Input: part model. Units: mm. Frame: model coordinates. Round coordinates to 2 decimals unless told otherwise and drop trailing zeros. Write each loop counter-clockwise with the first axis right and the second up, starting at its lowest first coordinate (ties: lowest second). Pieces come first, ordered by that corner, then holes. Notation, with made-up numbers: (-31, 52.25) - (11, 52.25) arc R18 ccw to (11, 71.25) - close; hole circle Ø5 at (-27.75, 23.25). An arc over 180 degrees is marked (long way). Use one line per item in the form item = value.
```python
from build123d import *

# Parameters (mm, degrees)
SKETCH_W        = 110
SKETCH_H        = 80
PAD_DEPTH       = 6
SKETCH001_R     = 1.4
POCKET_DEPTH    = 8
SKETCH002_R     = 2
POCKET001_DEPTH = 6


with BuildPart() as part:
    # Sketch → Pad (new body)
    with BuildSketch(Plane.XY):
        Rectangle(SKETCH_W, SKETCH_H)
    extrude(amount=PAD_DEPTH)

    # Sketch001 → Pocket (cut)
    with BuildSketch(Plane.XY.offset(6)):
        with Locations((-38.660252, 15)):
            Circle(SKETCH001_R)
        with Locations((-21.339748, -15)):
            Circle(SKETCH001_R)
        with Locations((-8.660252, 15)):
            Circle(SKETCH001_R)
        with Locations((8.660252, -15)):
            Circle(SKETCH001_R)
        with Locations((21.339748, 15)):
            Circle(SKETCH001_R)
        with Locations((38.660252, -15)):
            Circle(SKETCH001_R)
    extrude(amount=-POCKET_DEPTH, mode=Mode.SUBTRACT)

    # Sketch002 → Pocket001 (cut)
    with BuildSketch(Plane.XY.offset(6)):
        with Locations((-44.5, 32.1)):
            Circle(SKETCH002_R)
        with Locations((38.4, 32.1)):
            Circle(SKETCH002_R)
        with Locations((-30.4, 32.1)):
            Circle(SKETCH002_R)
        with Locations((-10.1, 32.1)):
            Circle(SKETCH002_R)
        with Locations((24.3, 32.1)):
            Circle(SKETCH002_R)
        with Locations((4, 32.1)):
            Circle(SKETCH002_R)
    pocket001 = extrude(amount=-POCKET001_DEPTH, mode=Mode.SUBTRACT)

    # Mirrored: Pocket001 across Sketch002 H_Axis
    add(pocket001.mirror(Plane(origin=(0, 0, 6), x_dir=(0, 0, 1), z_dir=(0, 1, 0))), mode=Mode.SUBTRACT)


solid = part.part
```
(1) Cut plane C-C on z = 3.4. Count the separate pieces of the cut face and the enclosed holes in it, then the cut area to 3 significant figures.
Derived:
separate_pieces = 1
enclosed_holes = 18
area = 8,610 mm^2
(2) Cut plane A-A on y = -15. Output: boundary loops of the cut face in (x, z).
Derived:
outline = (-55, 0) - (-22.74, 0) - (-22.74, 6) - (-55, 6) - close; (-19.94, 0) - (7.26, 0) - (7.26, 6) - (-19.94, 6) - close; (10.06, 0) - (37.26, 0) - (37.26, 6) - (10.06, 6) - close; (40.06, 0) - (55, 0) - (55, 6) - (40.06, 6) - close
(3) Material intervals for L1, parallel to Y at x = 38.4, z = 3.3; L2, parallel to Y at x = -44.5, z = 3.95; L3, parallel to Y at x = -43, z = 4.8, sorted ascending.
Derived:
L1 = -40 to -34.1, -30.1 to -16.38, -13.62 to 30.1, 34.1 to 40
L2 = -40 to -34.1, -30.1 to 30.1, 34.1 to 40
L3 = -40 to -33.42, -30.78 to 30.78, 33.42 to 40
(4) First-contact query: pin 1 Ø3.5 at (x, y) = (4, -32.1) entering from -Z. Flat tip, straight axial feed; report the tip coordinate or a pass-through.
Derived:
pin_1 = through
(5) Draft query along X for faces 1 (the face through (-55, -1, 3)), 2 (the face through (-1, 40, 3)), 3 (the face through (22.302, 32.188, 3.042)). Return one class per face: released by +X, released by -X, zero draft, split by the parting line, or undercut.
Derived:
face_1 = released by -X
face_2 = zero draft
face_3 = undercut
(6) Cut plane B-B on x = 4. Output: boundary loops of the cut face in (y, z), then the cut area to 3 significant figures.
Derived:
outline = (-40, 0) - (-34.1, 0) - (-34.1, 6) - (-40, 6) - close; (-30.1, 0) - (30.1, 0) - (30.1, 6) - (-30.1, 6) - close; (34.1, 0) - (40, 0) - (40, 6) - (34.1, 6) - close
area = 432 mm^2
(7) Cut plane D-D on x = 38.4. Output: boundary loops of the cut face in (y, z).
Derived:
outline = (-40, 0) - (-34.1, 0) - (-34.1, 6) - (-40, 6) - close; (-30.1, 0) - (-16.38, 0) - (-16.38, 6) - (-30.1, 6) - close; (-13.62, 0) - (30.1, 0) - (30.1, 6) - (-13.62, 6) - close; (34.1, 0) - (40, 0) - (40, 6) - (34.1, 6) - close
